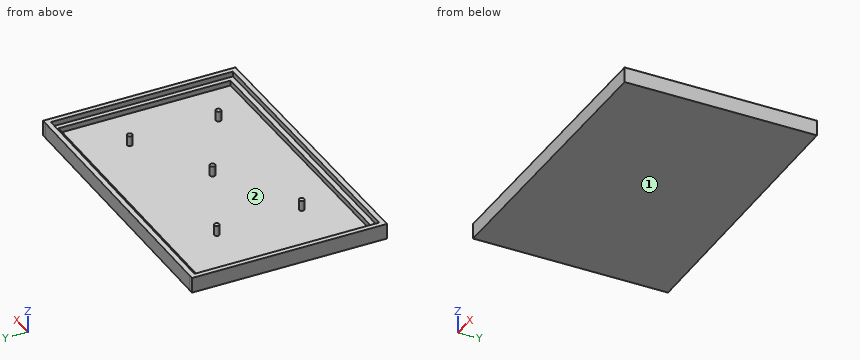
Solid Edge part; units mm, degrees
sketch "Sketch1" plane through (0, 0, 0) normal (0, 0, 1) x (1, 0, 0)
  line L0 (-23.4355, 0) -> (86.5645, 0)
  line L1 (86.5645, 0) -> (86.5645, 71)
  line L2 (-23.4309, 72) -> (86.5645, 71)
  line L3 (-23.4309, 72) -> (-23.4355, 0)
extrude "Protrusion1" add sketch "Sketch1" along normal blind 4
sketch "Sketch2" plane through (31.5645, 36, 4) normal (0, 0, 1) x (1, 0, 0)
  line L0 (-53, -34) -> (53, -34)
  line L1 (53, -34) -> (53, 33)
  line L2 (-52.9953, 34) -> (53, 33)
  line L3 (-52.9953, 34) -> (-53, -34)
extrude "ExtrudedCutout_1" cut sketch "Sketch2" against normal blind 2
sketch "Sketch3" plane through (31.5645, 36, 2) normal (0, 0, 1) x (-1, 0, 0)
  circle A0 centre (-35.0992, 20.046) radius 1
  circle A1 centre (-35.0992, -14.5315) radius 1
  circle A2 centre (-4.5458, 1.863) radius 1
  circle A3 centre (30.3299, -14.5315) radius 1
  circle A4 centre (29.4356, 19.046) radius 1
extrude "ExtrudedProtrusion_7" add sketch "Sketch3" along normal blind 4
sketch "Sketch4" plane through (0, 0, 0) normal (0, 0, 1) x (1, 0, 0)
  line L0 (-23.4309, 73.9825) -> (-23.4309, 74)
  line L1 (-23.4309, 74) -> (-25.4309, 74)
  line L2 (-25.4355, -2) -> (-25.4309, 74)
  line L3 (-23.4309, -2) -> (-25.4355, -2)
  line L4 (-23.4309, 72) -> (-23.4309, -2)
  line L5 (-23.4309, 72) -> (-23.4309, 73.9825)
extrude "ExtrudedProtrusion_8" add sketch "Sketch4" along normal blind 6
sketch "Sketch5" plane through (0, 0, 0) normal (0, 0, 1) x (1, 0, 0)
  line L0 (-23.4309, 0) -> (86.5645, 0)
  line L1 (86.5645, 0) -> (88.5645, 0)
  line L2 (88.5645, 0) -> (88.5645, -2)
  line L3 (88.5645, -2) -> (-23.4309, -2)
  line L4 (-23.4309, -2) -> (-23.4309, 0)
extrude "ExtrudedProtrusion_9" add sketch "Sketch5" along normal blind 6
sketch "Sketch6" plane through (0, 0, 0) normal (0, 0, 1) x (1, 0, 0)
  line L0 (86.5645, 0) -> (86.5645, 71)
  line L1 (86.5645, 71) -> (86.5645, 73)
  line L2 (86.5645, 73) -> (88.5645, 73)
  line L3 (88.5645, 73) -> (88.5645, 0)
  line L4 (88.5645, 0) -> (86.5645, 0)
extrude "ExtrudedProtrusion_10" add sketch "Sketch6" along normal blind 6
sketch "Sketch7" plane through (0, 0, 0) normal (0, 0, 1) x (1, 0, 0)
  line L0 (86.5645, 73) -> (86.5645, 71)
  line L1 (86.5645, 71) -> (-23.4309, 72)
  line L2 (-23.4309, 72) -> (-23.4309, 74)
  line L3 (-23.4309, 74) -> (86.5645, 73)
extrude "ExtrudedProtrusion_11" add sketch "Sketch7" along normal blind 6
Source: CAD feature listing. Evaluate the final solid. Frame: model axes, mm. Face numbers are marked on the shaded views. Give positions to 0.01 mm unless a question says otherwise; leave off trailing zeros. Order: outer loops, then holes, each group sorted by start corner. A loop starts at its lowest first (then second) coordinate and runs counter-clockwise, first axis right, second up.
(1) Section query B-B (x = 13.5). Return the cut outline in (y, z), plus the area to 3 significant figures.
(2) Section query C-C (y = 42). Return the cut outline in (x, z), plus the area to 3 significant figures.
(3) Section query A-A (z = 4.9). Return the cut outline in (x, y), plus the area to 3 significant figures.
(4) Pull-direction query (Y, two-part tool) for the marked faces 1 and 2; classes: +Y half, -Y half, draft (parallel to the pull), parting line (faces both ways), or undercut.
(5) Contact query for flat-ended pins moving along their axis: P1, Ø3, axis at x = 27.5, y = 16, coming from the +Z side; P2, Ø2, axis at x = 87.5, z = 2.5, coming from the +Y side; P3, Ø1.6, axis at x = 36.5, z = 5, coming from the +Y side. Output: stop coordinate, or through.
(6) Material intervals for line 1 along X through (y, z) = (17, 5.05); line 2 along X through (y, z) = (18, 3.1); line 3 along X through (y, z) = (54, 4.9), sorted ascending.
Outcome:
1. outline: (-2, 0) - (73.66, 0) - (73.66, 6) - (71.66, 6) - (71.66, 4) - (69.67, 4) - (69.67, 2) - (2, 2) - (2, 4) - (0, 4) - (0, 6) - (-2, 6) - close
1. area: 175 mm2
2. outline: (-25.43, 0) - (88.56, 0) - (88.56, 6) - (86.56, 6) - (86.56, 4) - (84.56, 4) - (84.56, 2) - (-21.43, 2) - (-21.43, 4) - (-23.43, 4) - (-23.43, 6) - (-25.43, 6) - close
2. area: 252 mm2
3. outline: (-25.44, -2) - (88.56, -2) - (88.56, 73) - (86.56, 73) - (-23.43, 74) - (-25.43, 74) - close; circle Ø2 at (1.23, 50.53); circle Ø2 at (2.13, 16.95); circle Ø2 at (36.11, 34.14); circle Ø2 at (66.66, 15.95); circle Ø2 at (66.66, 50.53); hole (-23.43, 0) - (86.56, 0) - (86.56, 71) - (-23.43, 72) - close
3. area: 758 mm2
4. face 1: draft
4. face 2: undercut
5. P1: stops at z = 2
5. P2: stops at y = 73
5. P3: stops at y = 73.46
6. line 1: x = -25.43 to -23.43, 1.13 to 3.13, 86.56 to 88.56
6. line 2: x = -25.43 to -21.43, 84.56 to 88.56
6. line 3: x = -25.43 to -23.43, 86.56 to 88.56
